Part model, mm, in its own coordinate system. Face numbers are marked on the shaded views. A direction names the side the tool comes from. Coordinates: 2 decimals unless noted, no trailing zeros. Loops run counter-clockwise (first coordinate to the right, second up) from the corner with the lowest first, then second, coordinate; pieces in that order, holes last. Notation, with made-up numbers: M 44,-20 L 66,-20 A18 cw 66,-2 Z; hole C 58,89 d8. An arc over 180 degrees is marked long. Answer as CSV lines item,"result". Start each with the question number.
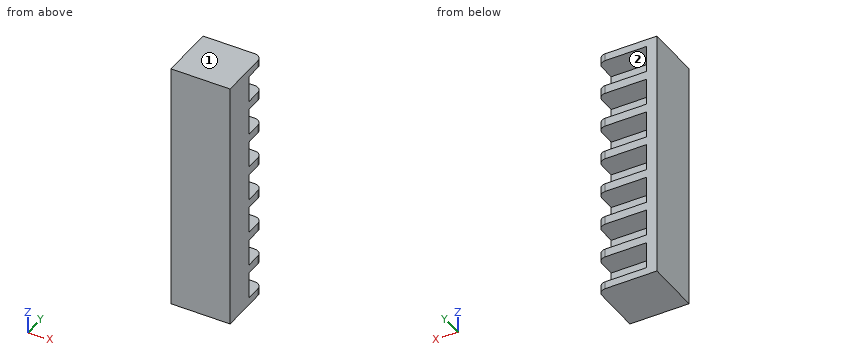
from build123d import *

# Parameters (mm, degrees)
SKETCH1_W           = 16
SKETCH1_H           = 68.25
BOSS_EXTRUDE1_DEPTH = 15
FILLET1_R           = 2
SKETCH2_W           = 13.2
SKETCH2_H           = 7.25
CUT_EXTRUDE1_DEPTH  = 6.25
LPATTERN1_COUNT     = 7
LPATTERN1_PITCH     = 9.5


with BuildPart() as part:
    # Sketch1 → Boss-Extrude1 (new body)
    with BuildSketch(Plane(origin=(0, 0, 0), x_dir=(1, 0, 0), z_dir=(0, 1, 0))):
        Rectangle(SKETCH1_W, SKETCH1_H)
    extrude(amount=BOSS_EXTRUDE1_DEPTH)

    # Fillet1
    fillet1_edges = [part.edges().sort_by_distance(p)[0] for p in [
        (8, 15, 0),
    ]]
    fillet(fillet1_edges, radius=FILLET1_R)

    # Sketch2 → Cut-Extrude1 (cut)
    with BuildSketch(Plane(origin=(0, 15, 0), x_dir=(1, 0, 0), z_dir=(0, 1, 0))):
        with Locations((1.4, -28.5)):
            Rectangle(SKETCH2_W, SKETCH2_H)
    cut_extrude1 = extrude(amount=-CUT_EXTRUDE1_DEPTH, mode=Mode.SUBTRACT)

    # LPattern1: Cut-Extrude1 ×7
    with Locations(*[(0, 0, -i * LPATTERN1_PITCH) for i in range(1, LPATTERN1_COUNT)]):
        add(cut_extrude1, mode=Mode.SUBTRACT)


solid = part.part
Q1. Slice it at C-C, the plane z = 1.5. Write the cut outline in (x, y).
Q2. Wall check: L1, parallel to X at y = 13, z = 9; L2, parallel to Y at x = 0.25, z = -1.5; L3, parallel to X at y = 14, z = -14.5. Give the ranges that are in metal, low to high.
Q3. Flat gauge pin, fed straight in: P1, Ø3, axis at y = 12, z = 18, coming from the +X side. Where does the tip first touch, or does it go through?
Q4. Tool access for the marked faces 1 and 2: list every direction of +Z, -Z, +X, -X, +Y, -Y with a clear straight run to the whole face (end or side of a thin tool).
Solved:
1,outline,"M -8,0 L 8,0 L 8,8.75 L -5.2,8.75 L -5.2,15 L -8,15 Z"
2,L1,"x = -8 to -5.2"
2,L2,"y = 0 to 8.75"
2,L3,"x = -8 to 7.73"
3,P1,"stops at x = -5.2"
4,face 1,"+Z, +X, -X, +Y, -Y"
4,face 2,"+X, +Y"
